Autodesk Inventor part; units mm, degrees
ref_plane "XZ Plane" through (0, 0, 0) normal (0, 1, 0) x (-1, 0, 0)
ref_plane "XY Plane" through (0, 0, 0) normal (0, 0, 1) x (1, 0, 0)
sketch "Sketch1" plane through (0, 0, 0) normal (0, 1, 0) x (-1, 0, 0)
  line L0 (28.575, 12.7) -> (-28.575, 12.7)
  line L1 (-28.575, 12.7) -> (-28.575, -12.7)
  line L2 (-28.575, -12.7) -> (28.575, -12.7)
  line L3 (28.575, -12.7) -> (28.575, 12.7)
  line L4 (28.575, 12.7) -> (-28.575, -12.7) construction
  line L5 (-28.575, 12.7) -> (28.575, -12.7) construction
  point P0 (0, 0)
  dimension "d0" = 57.15
  dimension "d1" = 25.4
extrude "Extrusion1" add sketch "Sketch1" against normal blind 6.35
sketch "Sketch2" plane through (0, 0, 0) normal (0, 1, 0) x (1, 0, 0)
  line L0 (-28.575, -12.7) -> (-28.575, 12.7)
  line L1 (-28.575, -12.7) -> (-22.225, -12.7)
  line L2 (-22.225, -12.7) -> (-22.225, 12.7)
  line L3 (-22.225, 12.7) -> (-28.575, 12.7)
  line L4 (-28.575, 12.7) -> (-28.575, -12.7)
  point P0 (0, 0)
  dimension "d4" = 6.35
extrude "Extrusion2" add sketch "Sketch2" along normal blind 215.9
sketch "Sketch5" plane through (-28.575, -6.35, -12.7) normal (-1, 0, 0) x (0, 0, 1)
  circle A0 centre (12.7, 19.05) radius 4.7625
  line L0 (0, 6.35) -> (25.4, 6.35)
  line L1 (12.7, 6.35) -> (12.7, 19.05) construction
  circle A1 centre (12.7, 66.675) radius 4.7625
  circle A2 centre (12.7, 114.3) radius 4.7625
  circle A3 centre (12.7, 161.925) radius 4.7625
  circle A4 centre (12.7, 209.55) radius 4.7625
  dimension "d33" = 9.525
  dimension "d34" = 12.7
  dimension "d37" = 47.625
extrude "Extrusion5" cut sketch "Sketch5" against normal through all
mirror "Mirror3" about plane through (0, 0, 0) normal (1, 0, 0) of "Extrusion2", "Extrusion5"
sketch "Sketch4" plane through (0, 0, 0) normal (0, 1, 0) x (1, 0, 0)
  point P0 (0, 0)
  point P1 (-12.7, 0)
  point P2 (12.7, 0)
  dimension "d24" = 12.7
  dimension "d25" = 12.7
hole "Hole1" at (-12.7, 0, 0) at (12.7, 0, 0) direction (0, -1, 0) diameter 5.6134 end through all
properties part number "camPostHolderV03"
The model under review builds one solid part; all positions refer to its coordinate system, in mm. A direction names the side the tool comes from. Round coordinates to 2 decimals unless told otherwise and drop trailing zeros. Loops run counter-clockwise (first coordinate to the right, second up) from the corner with the lowest first, then second, coordinate; pieces in that order, holes last. Notation, with made-up numbers: (-14.5, 56.5) -> (1.5, 56.5) arc R19 ccw to (1.5, 72.5) -> close; hole circle Ø4 at (44.25, 38.25). An arc over 180 degrees is marked (long way). Return JSON: item names as keys, results as strings.
(1) Add section C-C on y = 68. Write out the cut boundary in (x, z) (3 decimals).
Solved:
{"outline": "(-28.575, -12.7) -> (-22.225, -12.7) -> (-22.225, 12.7) -> (-28.575, 12.7) -> close; (22.225, -12.7) -> (28.575, -12.7) -> (28.575, 12.7) -> (22.225, 12.7) -> close"}
(2) Add section B-B on y = 203.2. Write out the cut boundary in (x, z) (1 decimal), plus the area to 3 significant figures.
Solved:
{"outline": "(-28.6, -12.7) -> (-22.2, -12.7) -> (-22.2, -4.8) -> (-28.6, -4.8) -> close; (-28.6, 4.8) -> (-22.2, 4.8) -> (-22.2, 12.7) -> (-28.6, 12.7) -> close; (22.2, -12.7) -> (28.6, -12.7) -> (28.6, -4.8) -> (22.2, -4.8) -> close; (22.2, 4.8) -> (28.6, 4.8) -> (28.6, 12.7) -> (22.2, 12.7) -> close", "area": "202 mm2"}
(3) For pin 1 (7.5 mm diameter, centred on x = -12.7, z = 0, fed in from +Y), flat-tipped, find the tip position at first contact; note if it passes through.
Solved:
{"pin 1": "y = 0"}
(4) Add section A-A on x = 12.7. Write out the cut boundary in (y, z), plus the area to 3 significant figures.
Solved:
{"outline": "(-6.35, -12.7) -> (0, -12.7) -> (0, -2.81) -> (-6.35, -2.81) -> close; (-6.35, 2.81) -> (0, 2.81) -> (0, 12.7) -> (-6.35, 12.7) -> close", "area": "126 mm2"}
(5) Add section D-D on z = -9.25. Write out the cut boundary in (x, y) (3 decimals), plus the area to 3 significant figures.
Solved:
{"outline": "(-28.575, -6.35) -> (28.575, -6.35) -> (28.575, 215.9) -> (22.225, 215.9) -> (22.225, 0) -> (-22.225, 0) -> (-22.225, 215.9) -> (-28.575, 215.9) -> close", "area": "3,100 mm2"}
(6) The part is to be moulded in two halves that separate along Z. For faces 3 (the flat face through (0, 0, 0)), 4 (the cylindrical face through (25.44, 198.48, -0.62)), 5 (the flat face through (-23, 88, 12.7)), say which applies: released by +Z, released by -Z, zero draft, split by the parting line, or undercut.
Solved:
{"face 3": "zero draft", "face 4": "undercut", "face 5": "released by +Z"}
(7) For line 1 (X direction, y = -1.75, z = 0) (3 decimals); line 2 (Y direction, x = -26, z = 0); line 3 (X direction, y = 93, z = 9) (3 decimals), list the stretches that pass through material, from the lowest coordinate up.
Solved:
{"line 1": "-28.575 to -15.507, -9.893 to 9.893, 15.507 to 28.575", "line 2": "-6.35 to 7.94, 17.46 to 55.56, 65.09 to 103.19, 112.71 to 150.81, 160.34 to 198.44, 207.96 to 215.9", "line 3": "-28.575 to -22.225, 22.225 to 28.575"}
(8) For faces 1 (the flat face through (-28.575, 106, 5)), 2 (the flat face through (22.225, 106, 5)), list the 3-axis set-ups (+Z, -Z, +X, -X, +Y, -Y) from which the entire face can be reached by the end or side of a thin tool; tool diameter is ignored.
Solved:
{"face 1": "+Z, -Z, -X, +Y, -Y", "face 2": "+Z, -Z, +Y"}
